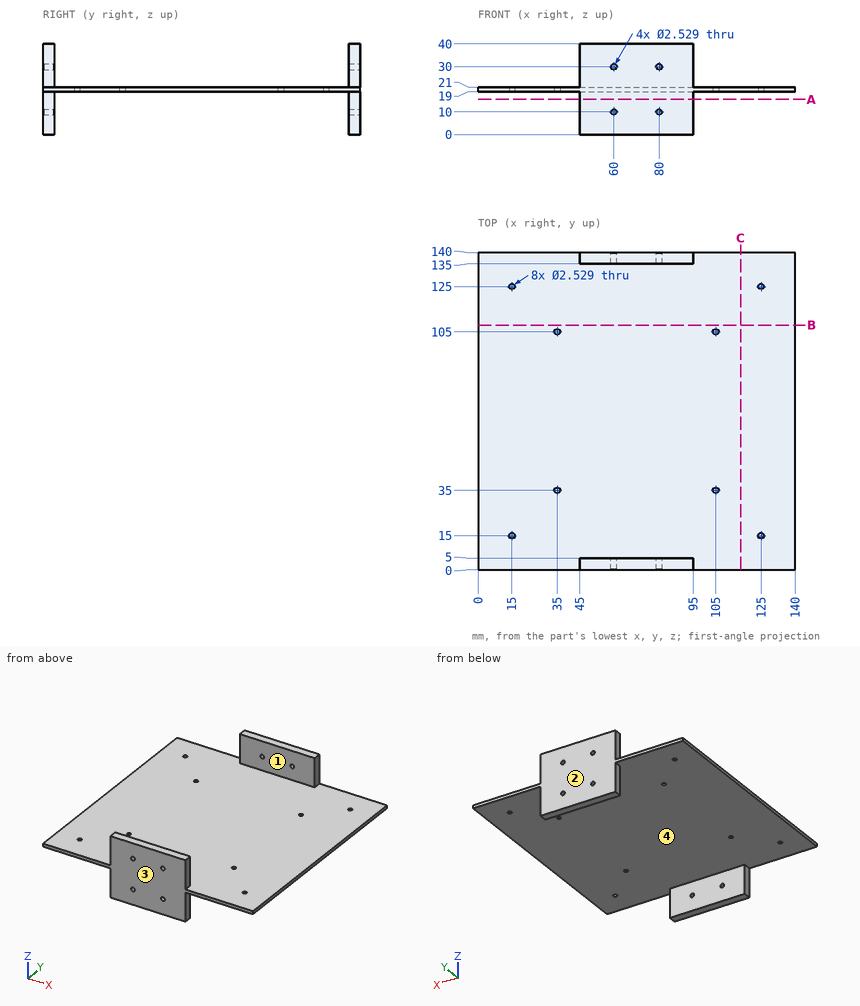
For this review, use the dimensioned drawing (mm, ordinates from the lowest corner) and the shaded views. Round coordinates to 2 decimals unless told otherwise and drop trailing zeros. Order: outer loops, then holes, each group sorted by start corner. A loop starts at its lowest first (then second) coordinate and runs counter-clockwise, first axis right, second up.
1) Consider section A-A (z = 15.5). State the section outline as (x, y) points.
The answers:
outline: (45, 0) - (95, 0) - (95, 5) - (45, 5) - close; (45, 135) - (95, 135) - (95, 140) - (45, 140) - close
2) Consider section B-B (y = 108). State the section outline as (x, z) points, plus the area to 3 significant figures.
The answers:
outline: (0, 19) - (140, 19) - (140, 21) - (0, 21) - close
area: 280 mm2
3) For L1, parallel to X at y = 136, z = 10; L2, parallel to Y at x = 62, z = 9.5; L3, parallel to Z at x = 60, y = 2.35, list the stretches that pass through material, from the lowest coordinate up.
The answers:
L1: x = 45 to 58.74, 61.26 to 78.74, 81.26 to 95
L2: y = 0 to 5, 135 to 140
L3: z = 0 to 8.74, 11.26 to 28.74, 31.26 to 40
4) Draft analysis for pull direction Y (two halves, no side actions). For the marked faces 1, 2, 3 and 4, state which applies: released by +Y, released by -Y, zero draft, split by the parting line, or undercut.
The answers:
face 1: undercut
face 2: released by +Y
face 3: released by -Y
face 4: undercut
5) Clearance check with flat-ended pins moving along their axes: pin 1 Ø8 at (x, y) = (123.5, 55) entering from +Z; pin 2 Ø2.5 at (y, z) = (2, 31.5) entering from -X; pin 3 Ø3.5 at (x, y) = (125, 125) entering from -Z. State where each tip first meets the part, or that it passes through.
The answers:
pin 1: stops at z = 21
pin 2: stops at x = 45
pin 3: stops at z = 19
